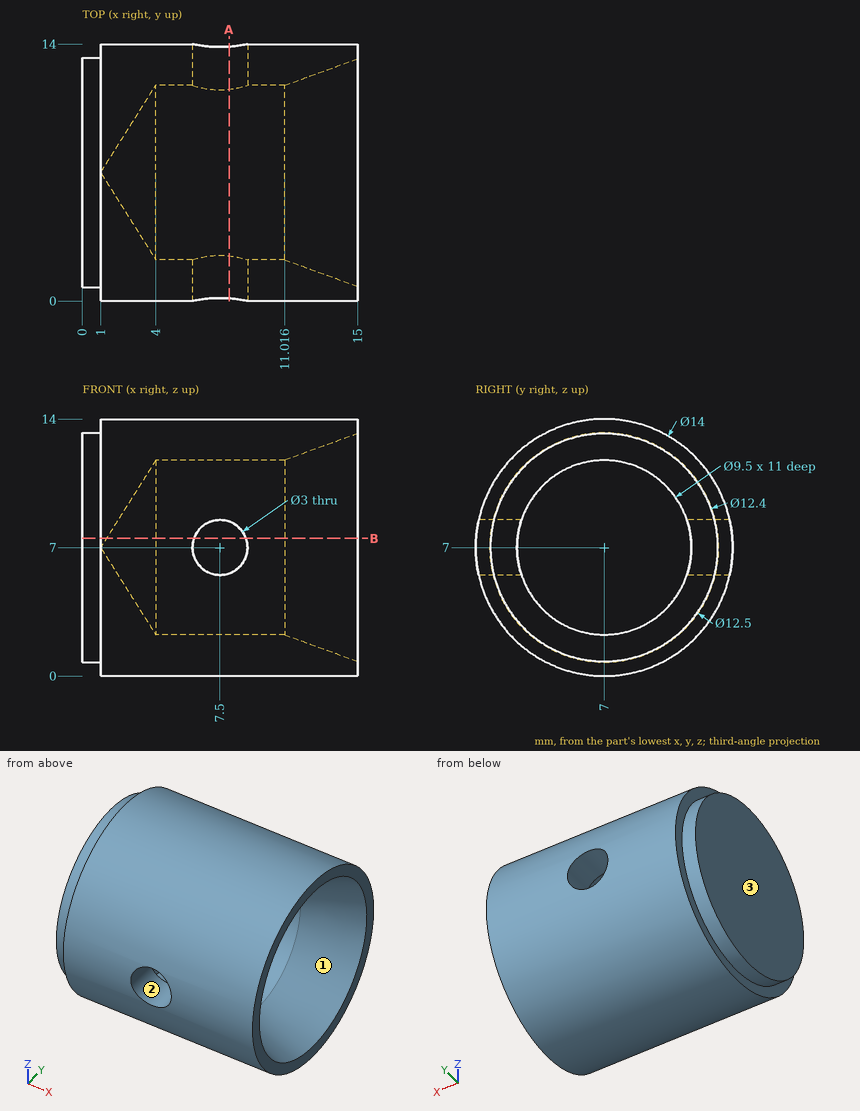
Geometry check sheet. Reference: drawing and pictorial views, mm from the part's lowest x, y, z. Give positions to 0.01 mm unless a question says otherwise; leave off trailing zeros. Order: outer loops, then holes, each group sorted by start corner. A loop starts at its lowest first (then second) coordinate and runs counter-clockwise, first axis right, second up. Notation, with made-up numbers: (15, 58) - (67, 58) arc R34 ccw to (67, 95) - close; hole circle Ø10 at (71, 5). An arc over 180 degrees is marked (long way). Use one line per item in the form item = value.
1) Material ranges on probe 1 along Y at (x, z) = (10, 8.25); probe 2 along Y at (x, z) = (11, 3.75) (1 decimal); probe 3 along Z at (x, y) = (7, 11) (1 decimal), recorded low to high. Write a range as from..to.
Working result:
probe_1 = 0.11..2.42, 11.58..13.89
probe_2 = 0.8..3.5, 10.5..13.2
probe_3 = 1.3..4.4, 9.6..12.7
2) Sectioned sample at B-B (z = 7.5). Count the separate pieces of the cut face and the enclosed holes in it.
Working result:
separate_pieces = 3
enclosed_holes = 0
3) Draft check along X on the marked faces 1, 2 and 3. Enter one of: released by +X, released by -X, zero draft, split by the parting line, or undercut.
Working result:
face_1 = released by +X
face_2 = undercut
face_3 = released by -X
4) Sectioned sample at A-A (x = 8). Record the boundary of the cut face in (y, z).
Working result:
outline = (0.14, 5.59) arc R7 ccw to (13.86, 5.59) - (11.53, 5.59) arc R4.75 cw to (2.47, 5.59) - close; (0.14, 8.41) - (2.47, 8.41) arc R4.75 cw to (11.53, 8.41) - (13.86, 8.41) arc R7 ccw to start
5) Depth check by flat-ended pin: pin 1 Ø1.5 at (x, z) = (3, 8.5) entering from -Y; pin 2 Ø2.5 at (x, z) = (7.5, 7) entering from +Y; pin 3 Ø3 at (y, z) = (6.5, 9.5) entering from +X; pin 4 Ø1.5 at (x, y) = (2.5, 2.5) entering from +Z. Enter the tip coordinate at first touch or a pass-through.
Working result:
pin_1 = 0.04
pin_2 = through
pin_3 = 3.56
pin_4 = 12.91
